Work out the finished part from the listing and answer in its coordinate system (mm). Face numbers are marked on the shaded views. A direction names the side the tool comes from. Round coordinates to 2 decimals unless told otherwise and drop trailing zeros. Write each loop counter-clockwise with the first axis right and the second up, starting at its lowest first coordinate (ties: lowest second). Pieces come first, ordered by that corner, then holes. Notation, with made-up numbers: M 2.25,74.5 L 51.25,74.5 A26 ccw 51.25,101.5 Z; hole C 19.25,26.25 d10. An arc over 180 degrees is marked long. Answer in a Markdown table with one row per item.
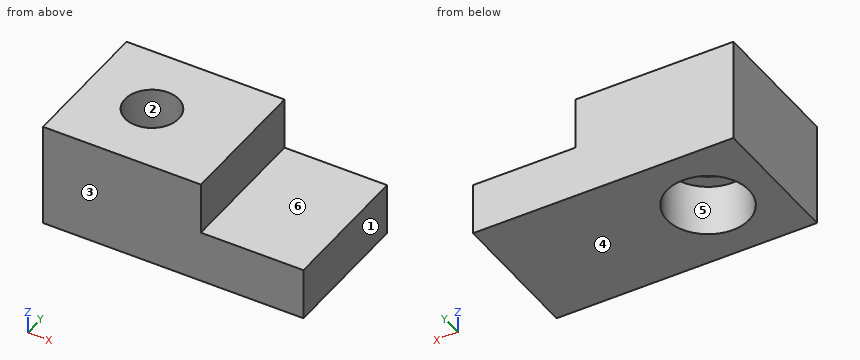
```python
from build123d import *

# Parameters (mm, degrees)
F0_W           = 25.4
F0_H           = 13.5920988396
F1_DEPTH       = 10.16
F2_D           = 5.25
F2_CBORE_D     = 8
F2_CBORE_DEPTH = 5
F3_W           = 10
F3_H           = 5.08
F4_DEPTH       = 25.4


with BuildPart() as f1:
    # F0 (on Top) → F1 (new body)
    with BuildSketch(Plane.XY):
        with Locations((12.7, 6.7960494198)):
            Rectangle(F0_W, F0_H)
    extrude(amount=F1_DEPTH)

    # F2 (through all)
    with Locations(Plane(origin=(0, 0, 0), x_dir=(1, 0, 0), z_dir=(0, 0, -1))):
        with Locations((6.5504941158, -6.7960494198)):
            CounterBoreHole(F2_D / 2, F2_CBORE_D / 2, F2_CBORE_DEPTH)

    # F3 (on face) → F4 (cut)
    with BuildSketch(Plane(origin=(0, 13.5920988396, 0), x_dir=(-1, 0, 0), z_dir=(0, 1, 0))):
        with Locations((-20.4, 7.62)):
            Rectangle(F3_W, F3_H)
    extrude(amount=-F4_DEPTH, mode=Mode.SUBTRACT)


solid = f1.part
```
1. The part is cut by section B-B (y = 1.25). Determine the outline of the cut face in (x, z).
Calculated:
| item | result |
|---|---|
| outline | M 0,0 L 25.4,0 L 25.4,5.08 L 15.4,5.08 L 15.4,10.16 L 0,10.16 Z |
2. Determine the mould class of the marked faces 1, 2 and 3 for opening direction X: released by +X, released by -X, zero draft, split by the parting line, or undercut.
Calculated:
| item | result |
|---|---|
| face 1 | released by +X |
| face 2 | undercut |
| face 3 | zero draft |
3. The part is cut by section A-A (x = 7.75). Determine the outline of the cut face in (y, z), plus the area to 3 significant figures.
Calculated:
| item | result |
|---|---|
| outline | M 0,0 L 2.98,0 L 2.98,5 L 4.46,5 L 4.46,10.16 L 0,10.16 Z; M 9.13,5 L 10.61,5 L 10.61,0 L 13.59,0 L 13.59,10.16 L 9.13,10.16 Z |
| area | 75.8 mm² |
4. A tool of negligible diameter and unlimited length cuts with its end or side. For the marked faces 4, 5 and 6, from which of +Z, -Z, +X, -X, +Y, -Y can it reach the whole face along a straight path? Write none if from no direction.
Calculated:
| item | result |
|---|---|
| face 4 | -Z, +X, -X, +Y, -Y |
| face 5 | -Z |
| face 6 | +Z, +X, +Y, -Y |
5. Consider line 1 along X through (y, z) = (7, 2); line 2 along X through (y, z) = (5.5, 6); line 3 along Y through (x, z) = (3.75, 3.75). Determine where each line is inside the solid, lowest interval first. Write a range as from..to.
Calculated:
| item | result |
|---|---|
| line 1 | x = 0..2.56, 10.55..25.4 |
| line 2 | x = 0..4.27, 8.83..15.4 |
| line 3 | y = 0..3.94, 9.65..13.59 |
6. The part is cut by section D-D (x = 4.75). Determine the outline of the cut face in (y, z), plus the area to 3 significant figures.
Calculated:
| item | result |
|---|---|
| outline | M 0,0 L 3.22,0 L 3.22,5 L 4.89,5 L 4.89,10.16 L 0,10.16 Z; M 8.71,5 L 10.37,5 L 10.37,0 L 13.59,0 L 13.59,10.16 L 8.71,10.16 Z |
| area | 82.7 mm² |
7. Given pin 1 (2 mm diameter, centred on y = 6, z = 5, fed in from -X); pin 2 (3 mm diameter, centred on x = 22, y = 9.5, fed in from +Z); pin 3 (2 mm diameter, centred on y = 9.5, z = 8.5, fed in from +X), each flat-ended and moving along its own axis, determine where each tip first touches the part or whether it passes through.
Calculated:
| item | result |
|---|---|
| pin 1 | stops at x = 0 |
| pin 2 | stops at z = 5.08 |
| pin 3 | stops at x = 15.4 |
